from build123d import *

# Parameters (mm, degrees)
BOSS_EXTRUDE1_DEPTH = 2
SKETCH2_W           = 67
SKETCH2_H           = 43
BOSS_EXTRUDE2_DEPTH = 13
SKETCH3_R           = 2
CUT_EXTRUDE1_DEPTH  = 3.0000001
FILLET1_R           = 6
FILLET2_R           = 1


with BuildPart() as part:
    # Sketch1 → Boss-Extrude1 (new body)
    with BuildSketch(Plane(origin=(0, 0, 0), x_dir=(1, 0, 0), z_dir=(0, 1, 0))):
        with BuildLine():
            Line((85, 0), (10, 0))
            add(Edge.make_bspline(
                [(10, 0), (7e-09, -10.749999992), (0, -21.499999985)],
                knots=[0, 0, 0, 0.5, 0.5, 0.5], degree=2))
            add(Edge.make_bspline(
                [(0, -21.499999985), (-7e-09, -32.249999992), (10, -43)],
                knots=[0.5, 0.5, 0.5, 1, 1, 1], degree=2))
            Line((10, -43), (85, -43))
            Line((85, -43), (85, 0))
        make_face()
    extrude(amount=BOSS_EXTRUDE1_DEPTH)

    # Sketch2 → Boss-Extrude2 (add)
    with BuildSketch(Plane(origin=(0, 2, 0), x_dir=(1, 0, 0), z_dir=(0, 1, 0))):
        with Locations((43.5, -21.5)):
            Rectangle(SKETCH2_W, SKETCH2_H)
    extrude(amount=BOSS_EXTRUDE2_DEPTH)

    # Sketch3 → Cut-Extrude1 (cut, through all)
    with BuildSketch(Plane(origin=(0, 2, 0), x_dir=(1, 0, 0), z_dir=(0, 1, 0))):
        with Locations((80, -5)):
            Circle(SKETCH3_R)
        with Locations((80, -38)):
            Circle(SKETCH3_R)
        with Locations((5, -21.500000001)):
            Circle(SKETCH3_R)
    extrude(amount=-CUT_EXTRUDE1_DEPTH, mode=Mode.SUBTRACT)

    # Fillet1
    fillet1_edges = [part.edges().sort_by_distance(p)[0] for p in [
        (85, 1, 0),
        (85, 1, 43),
    ]]
    fillet(fillet1_edges, radius=FILLET1_R)

    # Fillet2
    fillet2_edges = [part.edges().sort_by_distance(p)[0] for p in [
        (77, 8.5, 43),
        (77, 8.5, 0),
        (10, 15, 21.5),
        (43.5, 15, 43),
        (77, 15, 21.5),
        (43.5, 15, 0),
    ]]
    fillet(fillet2_edges, radius=FILLET2_R)


solid = part.part
Part model, mm, in its own coordinate system. A direction names the side the tool comes from. Give positions to 0.01 mm unless a question says otherwise; leave off trailing zeros. Loops run counter-clockwise (first coordinate to the right, second up) from the corner with the lowest first, then second, coordinate; pieces in that order, holes last.
(1) Band-saw the part on C-C (y = 1). Count the separate pieces of the cut face and the enclosed holes in it, and give its area (3 significant figures).
Return value:
separate pieces: 1
enclosed holes: 3
area: 3,460 mm2
(2) 3-axis set-ups, long thin cutter, end or side, ignore diameter. For faces 4 (the cylindrical face through (3.526, 1.014, 20.148)), 5 (the flat face through (77, 8, 22)), 6 (the flat face through (7, 2, 23)): which of +Z, -Z, +X, -X, +Y, -Y reach the whole face in a straight line?
Return value:
face 4: +Y, -Y
face 5: +Z, -Z, +X, +Y
face 6: +Z, -Z, -X, +Y
(3) Band-saw the part on B-B (y = 4.5). Write the cut outline in (x, z).
Return value:
outline: (10, 0) - (76, 0) arc R1 ccw to (77, 1) - (77, 42) arc R1 ccw to (76, 43) - (10, 43) - close
(4) Pull direction Z, two halves, no side cores. Call faces 1 (the flat face through (10, 8, 22)), 2 (the flat face through (44, 7, 43)), 3 (the cylindrical face through (81.908, 1.014, 4.399)): pulls with the +Z half, pulls with the -Z half, needs draft (parallel to the pull), parting line crosses it, or undercut.
Return value:
face 1: needs draft
face 2: pulls with the +Z half
face 3: undercut
(5) Drill centre lines: line 1 along Z through (x, y) = (80, 1.05); line 2 along X through (y, z) = (9.5, 7); line 3 along Y through (x, z) = (9, 35). Where is each one in solid material? Low to high.
Return value:
line 1: z = 0.08 to 3, 7 to 36, 40 to 42.92
line 2: x = 10 to 77
line 3: y = 0 to 2
(6) Band-saw the part on A-A (x = 80). Write the cut outline in (y, z), and give its area (3 significant figures).
Return value:
outline: (0, 0.08) - (2, 0.08) - (2, 3) - (0, 3) - close; (0, 7) - (2, 7) - (2, 36) - (0, 36) - close; (0, 40) - (2, 40) - (2, 42.92) - (0, 42.92) - close
area: 69.7 mm2
(7) Pin check, flat tips, straight feed: pin 1 (6 mm diameter, centred on y = 6.5, z = 31.5, fed in from +X); pin 2 (11 mm diameter, centred on x = 3.5, z = 16, fed in from +Y); pin 3 (3 mm diameter, centred on x = 5, z = 21.5, fed in from -Y); pin 4 (6 mm diameter, centred on y = 5.5, z = 24, fed in from -X). Stop position of each tip, or through.
Return value:
pin 1: stops at x = 77
pin 2: stops at y = 2
pin 3: passes through
pin 4: stops at x = 10
